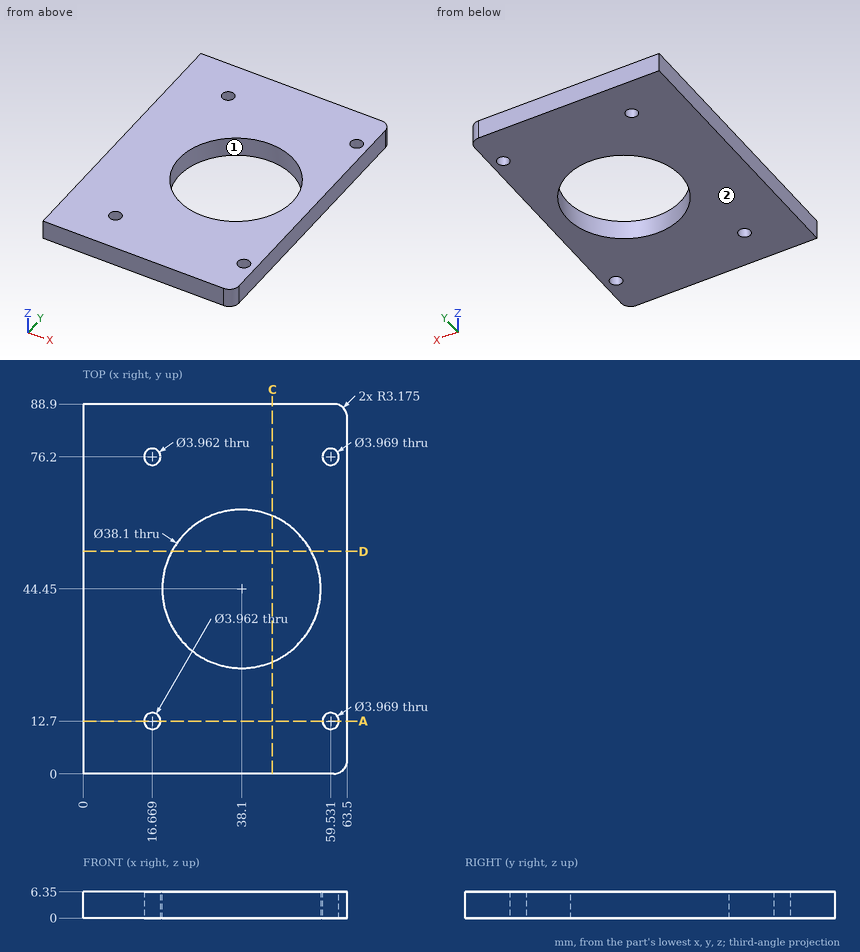
Can you work these out from the drawing? Everything is in mm from the part's minimum corner. Round coordinates to 2 decimals unless told otherwise and drop trailing zeros. Order: outer loops, then holes, each group sorted by start corner. A loop starts at its lowest first (then second) coordinate and runs counter-clockwise, first axis right, second up. Notation, with made-up numbers: M 6.5,7.5 L 45.5,7.5 A21 ccw 45.5,11.5 Z; hole C 23,19.5 d9. An arc over 180 degrees is marked long. One line per question, with ' | ' between items.
1) I want a section at A-A, the plane y = 12.7. State how many separate pieces and enclosed holes the cut face has, then the cut area to 3 significant figures.
Working result:
separate pieces: 3 | enclosed holes: 0 | area: 353 mm²
2) For pin 1 Ø3 at (x, y) = (59.53, 76.2) entering from -Z, with a flat end and sliding along its axis, tell me the tip position at first contact or that it passes through.
Working result:
pin 1: through
3) I need wall thicknesses on line 1 along Y through (x, z) = (59.5, 1) (1 decimal); line 2 along X through (y, z) = (44.5, 3); line 3 along Y through (x, z) = (58, 1) (1 decimal). Which ranges of each line are inside material? Lowest first, please.
Working result:
line 1: 0 to 10.7, 14.7 to 74.2, 78.2 to 88.9 | line 2: 0 to 19.05, 57.15 to 63.5 | line 3: 0 to 11.4, 14 to 74.9, 77.5 to 88.9
4) I want a section at C-C, the plane x = 45.5. Write out the boundary of the cut face in (y, z).
Working result:
outline: M 0,0 L 26.9,0 L 26.9,6.35 L 0,6.35 Z; M 62,0 L 88.9,0 L 88.9,6.35 L 62,6.35 Z
5) I want a section at D-D, the plane y = 53.5. Write out the boundary of the cut face in (x, z).
Working result:
outline: M 0,0 L 21.34,0 L 21.34,6.35 L 0,6.35 Z; M 54.86,0 L 63.5,0 L 63.5,6.35 L 54.86,6.35 Z
6) If we mould it in two halves opening along Y, with no side actions, what happens to the marked faces 1 and 2? For each: +Y half, -Y half, draft (parallel to the pull), parting line (faces both ways), or undercut.
Working result:
face 1: undercut | face 2: draft
